```python
from build123d import *

# Parameters (mm, degrees)
SKETCH1_W           = 17
SKETCH1_H           = 14
SKETCH1_W_2         = 9
SKETCH1_H_2         = 9
SKETCH1_W_3         = 6
SKETCH1_H_3         = 6
BOSS_EXTRUDE1_DEPTH = 4.8
CUT_EXTRUDE1_START  = -4.8
SKETCH1_6_W         = 9
SKETCH1_6_H         = 9
SKETCH1_6_W_2       = 6
SKETCH1_6_H_2       = 6
CUT_EXTRUDE1_DEPTH  = 3
SKETCH1_3_W         = 6
SKETCH1_3_H         = 6
BOSS_EXTRUDE2_DEPTH = 5.5


with BuildPart() as part:
    # Sketch1 → Boss-Extrude1 (new body)
    # profile 1 of 3: a face of its own
    with BuildSketch(Plane(origin=(0, 0, 0), x_dir=(1, 0, 0), z_dir=(0, 1, 0))):
        Rectangle(SKETCH1_W, SKETCH1_H)
        Rectangle(SKETCH1_W_2, SKETCH1_H_2, mode=Mode.SUBTRACT)
    # profile 2 of 3: a face of its own
    with BuildSketch(Plane(origin=(0, 0, 0), x_dir=(1, 0, 0), z_dir=(0, 1, 0))):
        Rectangle(SKETCH1_W_2, SKETCH1_H_2)
        Rectangle(SKETCH1_W_3, SKETCH1_H_3, mode=Mode.SUBTRACT)
    # profile 3 of 3: a face of its own
    with BuildSketch(Plane(origin=(0, 0, 0), x_dir=(1, 0, 0), z_dir=(0, 1, 0))):
        Rectangle(SKETCH1_W_3, SKETCH1_H_3)
    extrude(amount=-BOSS_EXTRUDE1_DEPTH)

    # Sketch1_6 → Cut-Extrude1 (cut)
    # profile 1 of 2: a face of its own
    with BuildSketch(Plane(origin=(0, 0, 0), x_dir=(1, 0, 0), z_dir=(0, 1, 0)).offset(CUT_EXTRUDE1_START)):
        Rectangle(SKETCH1_6_W, SKETCH1_6_H)
        Rectangle(SKETCH1_6_W_2, SKETCH1_6_H_2, mode=Mode.SUBTRACT)
    # profile 2 of 2: a face of its own
    with BuildSketch(Plane(origin=(0, 0, 0), x_dir=(1, 0, 0), z_dir=(0, 1, 0)).offset(CUT_EXTRUDE1_START)):
        Rectangle(SKETCH1_6_W_2, SKETCH1_6_H_2)
    extrude(amount=CUT_EXTRUDE1_DEPTH, mode=Mode.SUBTRACT)

    # Sketch1_3 → Boss-Extrude2 (add)
    with BuildSketch(Plane(origin=(0, 0, 0), x_dir=(1, 0, 0), z_dir=(0, 1, 0))):
        Rectangle(SKETCH1_3_W, SKETCH1_3_H)
    extrude(amount=BOSS_EXTRUDE2_DEPTH)


solid = part.part
```
Input: part model. Units: mm. Frame: model coordinates. A direction names the side the tool comes from. Give positions to 0.01 mm unless a question says otherwise; leave off trailing zeros. Loops run counter-clockwise (first coordinate to the right, second up) from the corner with the lowest first, then second, coordinate; pieces in that order, holes last. Notation, with made-up numbers: M 7,38 L 48,38 A10 cw 48,44 Z; hole C -23,20.25 d9. An arc over 180 degrees is marked long. Answer as CSV lines item,"result". Start each with the question number.
1. Pin query (flat end, axial travel): P1, Ø2, axis at y = 1.5, z = -1, coming from the +X side; P2, Ø2, axis at y = 2.5, z = -2, coming from the -X side; P3, Ø1.5, axis at x = 3, z = 4, coming from the +Y side; P4, Ø8, axis at x = 1.5, z = -5.5, coming from the +Y side. Return the tip coordinate at first contact, or that it passes through.
2. Pull-direction query (Z, two-part tool) for faces 1 (the face through (0, -2, 7)), 2 (the face through (0, -4.8, -5)), 3 (the face through (0, -3, -4.5)); classes: released by +Z, released by -Z, zero draft, split by the parting line, or undercut.
3. Section D-D on y = 2.25. Return loops of the section in (x, z).
4. Reachability of faces 4 (the face through (0, -1.8, 0)), 5 (the face through (0, 3, 3)), 6 (the face through (0, 3, -3)), 7 (the face through (3, 3, 0)) from +Z, -Z, +X, -X, +Y, -Y: full face, straight path, thin tool, end or side. Return the list, or none.
5. Section C-C on x = -0.25. Return loops of the section in (y, z), plus the area to 3 significant figures.
6. Section B-B on z = -2. Return loops of the section in (x, y).
7. Line query: L1, parallel to Z at x = 3.25, y = -3.25; L2, parallel to X at y = -2.5, z = -3.5; L3, parallel to X at y = 0.25, z = 0.5. Output: solid intervals per line, ascending.
8. Section A-A on y = -2.25. Return loops of the section in (x, z).
Computed values:
1,P1,"stops at x = 3"
1,P2,"stops at x = -3"
1,P3,"stops at y = 0"
1,P4,"stops at y = 5.5"
2,face 1,"released by +Z"
2,face 2,"zero draft"
2,face 3,"undercut"
3,outline,"M -3,-3 L 3,-3 L 3,3 L -3,3 Z"
4,face 4,"-Y"
4,face 5,"+Z, +X, -X, +Y"
4,face 6,"-Z, +X, -X, +Y"
4,face 7,"+Z, -Z, +X, +Y"
5,outline,"M -4.8,-7 L 0,-7 L 0,-3 L 5.5,-3 L 5.5,3 L 0,3 L 0,7 L -4.8,7 L -4.8,4.5 L -1.8,4.5 L -1.8,-4.5 L -4.8,-4.5 Z"
5,area,"73.2 mm²"
6,outline,"M -8.5,-4.8 L -4.5,-4.8 L -4.5,-1.8 L 4.5,-1.8 L 4.5,-4.8 L 8.5,-4.8 L 8.5,0 L 3,0 L 3,5.5 L -3,5.5 L -3,0 L -8.5,0 Z"
7,L1,"z = -7 to -4.5, 4.5 to 7"
7,L2,"x = -8.5 to -4.5, 4.5 to 8.5"
7,L3,"x = -3 to 3"
8,outline,"M -8.5,-7 L 8.5,-7 L 8.5,7 L -8.5,7 Z; hole M -4.5,-4.5 L 4.5,-4.5 L 4.5,4.5 L -4.5,4.5 Z"
